from build123d import *

# Parameters (mm, degrees)
F6_DEPTH  = 166.5272102769
F9_DEPTH  = 101.6
F10_DEPTH = 39.8337877091
F12_W     = 2.54
F12_H     = 2.54
F13_DEPTH = 25.4
F14_DEPTH = 12.7
F15_R     = 22.225
F16_DEPTH = 2.54


# Not quite as in the source:
# - the program builds the solid bodies; features that only make, move or delete a surface that nothing else refers to are left out


with BuildPart() as f3:
    # F0 (on Top) → F3 section 0
    with BuildSketch(Plane.XY, mode=Mode.PRIVATE) as f3_s0:
        Polygon((115.7262101769, -133.7715089321), (0, 192.2327876091), (-115.7262101769, -133.7715089321), (-38.9538705349, -89.2658084631), (-70.1078623533, -133.7715089321), (-18.8981407312, -104.0847162377), (0, -202.7553617954), (18.8981407312, -104.0847162377), (70.1078623533, -133.7715089321), (38.9538705349, -89.2658084631), align=None)
    loft([f3_s0.sketch, Vertex(0, 60.7637315989, 25.4)])

    # F5 (on offset) → F6 (cut, through all)
    with BuildSketch(Plane.YZ.offset(50.8)):
        Polygon((94.1726788878, 13.6528518051), (60.1693615317, 19.8352746665), (36.985270679, 5.446716453), (92.6806539106, 5.446716453), align=None)
    extrude(amount=-F6_DEPTH, mode=Mode.SUBTRACT)

    # F8 (on offset) → F9 (cut)
    with BuildSketch(Plane.XZ.offset(-152.4)):
        Polygon((-12.4854929745, 5.5678542703), (11.810598895, 5.5678542703), (4.7242408618, 11.641876772), (0, 21.0903566331), (-5.3991349414, 11.641876772), align=None)
    extrude(amount=F9_DEPTH, mode=Mode.SUBTRACT)

    # F10 (cut, through all): a face of the model
    f10_faces = [f3.faces().sort_by_distance(p)[0] for p in [
        (0, 152.4, 6.2771523841),
    ]]
    extrude(f10_faces, amount=-F10_DEPTH, mode=Mode.SUBTRACT)

    # F12 (on offset) → F13 (join)
    with BuildSketch(Plane.XZ.offset(-127)):
        with Locations((17.467392717, 4.4757343051)):
            Rectangle(F12_W, F12_H)
        with Locations((-17.467392717, 4.4757343051)):
            Rectangle(F12_W, F12_H)
    extrude(amount=F13_DEPTH)

    # F14 (cut): faces of the model
    f14_faces = [f3.faces().sort_by_distance(p)[0] for p in [
        (17.5136661011, 127, 4.5302328808),
        (-17.5136661011, 127, 4.5302328808),
    ]]
    extrude(f14_faces, amount=-F14_DEPTH, mode=Mode.SUBTRACT)

    # F15 (on face) → F16 (cut)
    with BuildSketch(Plane(origin=(0, 0, 0), x_dir=(1, 0, 0), z_dir=(0, 0, -1))):
        with Locations((-51.2486876787, 53.3265663744)):
            Circle(F15_R)
        with Locations((51.2486876787, 53.3265663744)):
            Circle(F15_R)
        with Locations((0, 0.0474439003)):
            Circle(F15_R)
        with Locations((0, -88.4402606044)):
            Circle(F15_R)
    extrude(amount=-F16_DEPTH, mode=Mode.SUBTRACT)


solid = f3.part
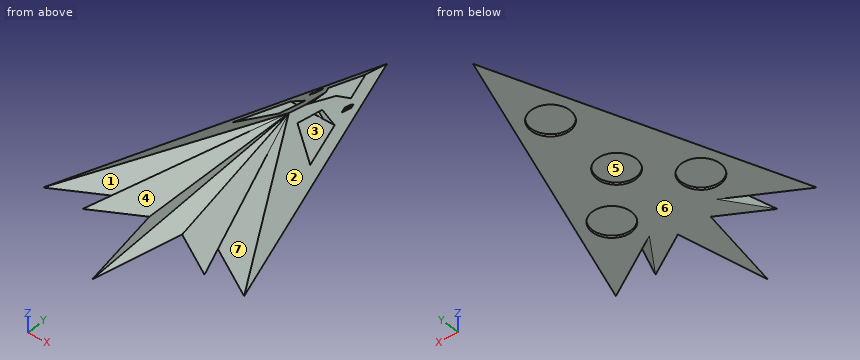
The model under review builds one solid part; all positions refer to its coordinate system, in mm. Face numbers are marked on the shaded views. A direction names the side the tool comes from. Coordinates: 2 decimals unless noted, no trailing zeros. Write each loop counter-clockwise with the first axis right and the second up, starting at its lowest first coordinate (ties: lowest second). Pieces come first, ordered by that corner, then holes. Notation, with made-up numbers: (88, 31) - (115, 31) arc R10 ccw to (115, 46) - close; hole circle Ø11 at (-25, -14). An arc over 180 degrees is marked (long way). Answer as a JSON object with one key per item and string values. Group by question number.
1. Machinability: for the marked faces 4, 5, 6 and 7, which of the approach directions +Z, -Z, +X, -X, +Y, -Y give a long, thin tool a straight path to every point of the face, cutting with its end or side? Answer none if there is none.
2. Add section D-D (y = -176.5). Give the boundary of the cut face in (x, z), plus the area to 3 significant figures.
3. Mouldability with a two-part tool opening along X and no side actions: class the marked faces 1, 2 and 3 as pulls with the +X half, pulls with the -X half, needs draft (parallel to the pull), parting line crosses it, or undercut.
4. To check wall thickness, follow probe 1 along Z at (x, y) = (65, -101); probe 2 along Z at (x, y) = (-23, 43); probe 3 along Z at (x, y) = (-82, -80). State the ranges of each line that lie inside material, in increasing order.
5. Add section A-A (y = 70.5). Give the boundary of the cut face in (x, z).
6. Add section C-C (y = -98). Give the boundary of the cut face in (x, z), plus the area to 3 significant figures.
7. Add section B-B (x = 49). Give the boundary of the cut face in (y, z), plus the area to 3 significant figures.
8. Clearance check with flat-ended pins moving along their axes: pin 1 Ø2 at (x, z) = (-33, 20.5) entering from +Y; pin 2 Ø1.3 at (x, z) = (-17.5, 4.5) entering from +Y; pin 3 Ø0.8 at (x, y) = (-17.5, 111.5) entering from +Z; pin 4 Ø22 at (x, y) = (-7.5, -0.5) entering from -Z. State where each tip first meets the part, or that it passes through.
Findings:
{
 "1": {"face 4": "+Z, -Y", "face 5": "-Z", "face 6": "-Z, +X, -X, +Y, -Y", "face 7": "none"},
 "2": {"outline": "(-5.03, 0) - (5.03, 0) - (0, 2.53) - close", "area": "12.7 mm²"},
 "3": {"face 1": "undercut", "face 2": "pulls with the +X half", "face 3": "needs draft"},
 "4": {"probe 1": "0 to 0.67", "probe 2": "0 to 5.45, 9.18 to 16.31", "probe 3": "0 to 6.82"},
 "5": {"outline": "(-43.21, 0) - (-13.12, 0) - (-13.12, 2.54) - (13.12, 2.54) - (13.12, 0) - (43.21, 0) - (33.21, 5.45) - (-33.21, 5.45) - close; (-10.22, 17.96) - (-1.79, 17.96) - (0, 21.09) - (1.57, 17.96) - (10.22, 17.96) - (0, 23.52) - close"},
 "6": {"outline": "(-103.03, 0) - (-54.02, 0) - (-94.45, 4.67) - close; (-57.22, 4.67) - (-45.07, 0) - (45.07, 0) - (57.22, 4.67) - (18.2, 0.94) - (0, 10.1) - (-18.2, 0.94) - close; (54.02, 0) - (103.03, 0) - (94.45, 4.67) - close", "area": "592 mm²"},
 "7": {"outline": "(-121.54, 0) - (-103.62, 0) - (-75.2, 7.65) - close; (-95.09, 0) - (-75.44, 0) - (-75.44, 2.54) - (-31.22, 2.54) - (-31.22, 0) - (54.2, 0) - (-21.61, 14.65) - close", "area": "1,050 mm²"},
 "8": {"pin 1": "through", "pin 2": "y = 114.3", "pin 3": "z = 6.3", "pin 4": "z = 2.54"}
}
